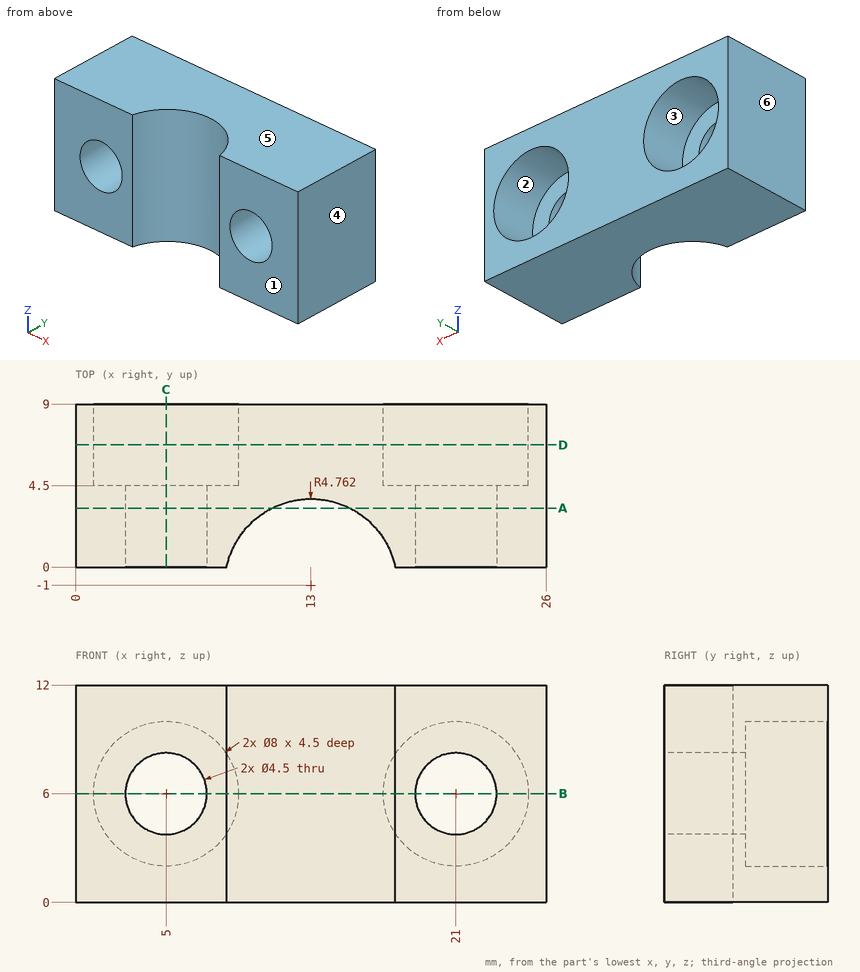
For this review, use the dimensioned drawing (mm, ordinates from the lowest corner) and the shaded views. A direction names the side the tool comes from. Round coordinates to 2 decimals unless told otherwise and drop trailing zeros. Write each loop counter-clockwise with the first axis right and the second up, starting at its lowest first coordinate (ties: lowest second). Pieces come first, ordered by that corner, then holes. Notation, with made-up numbers: (75, 57.25) - (105, 57.25) arc R13 ccw to (105, 76.25) - close; hole circle Ø10 at (73.25, 39). An arc over 180 degrees is marked (long way). Answer as CSV lines item,"result". Start each with the question number.
(1) We need section D-D on y = 6.75. State the section outline as (x, z) points.
(2) Draft analysis for pull direction X (two halves, no side actions). For the marked faces 3, 4, 5 and 6, state which applies: pulls with the +X half, pulls with the -X half, needs draft (parallel to the pull), parting line crosses it, or undercut.
(3) We need section C-C on x = 5. State the section outline as (y, z) points.
(4) To check wall thickness, follow line 1 (Z direction, x = 5, y = 6.2); line 2 (X direction, y = 3, z = 11) (1 decimal); line 3 (X direction, y = 6.25, z = 6.5). State the ranges of each line that lie inside material, in increasing order.
(5) We need section B-B on z = 6. Give the number of separate pieces and of enclosed holes in the cut face.
(6) We need section A-A on y = 3.25. State the section outline as (x, z) points.
(7) For pin 1 Ø5 at (x, z) = (5, 6) entering from +Y, flat-tipped, find the tip position at first contact; note if it passes through.
(8) For the marked faces 1 and 2, list the 3-axis set-ups (+Z, -Z, +X, -X, +Y, -Y) from which the entire face can be reached by the end or side of a thin tool; tool diameter is ignored.
Worked answers:
1,outline,"(0, 0) - (26, 0) - (26, 12) - (0, 12) - close; hole circle Ø8 at (5, 6); hole circle Ø8 at (21, 6)"
2,face 3,"undercut"
2,face 4,"pulls with the +X half"
2,face 5,"needs draft"
2,face 6,"pulls with the -X half"
3,outline,"(0, 0) - (9, 0) - (9, 2) - (4.5, 2) - (4.5, 3.75) - (0, 3.75) - close; (0, 8.25) - (4.5, 8.25) - (4.5, 10) - (9, 10) - (9, 12) - (0, 12) - close"
4,line 1,"0 to 2, 10 to 12"
4,line 2,"0 to 10.4, 15.6 to 26"
4,line 3,"0 to 1.03, 8.97 to 17.03, 24.97 to 26"
5,separate pieces,"3"
5,enclosed holes,"0"
6,outline,"(0, 0) - (10.85, 0) - (10.85, 12) - (0, 12) - close; (15.15, 0) - (26, 0) - (26, 12) - (15.15, 12) - close; hole circle Ø4.5 at (5, 6); hole circle Ø4.5 at (21, 6)"
7,pin 1,"y = 4.5"
8,face 1,"+Z, -Z, +X, -X, -Y"
8,face 2,"+Y"
